Part print with two shaded views. Sizes in mm from the minimum x, y, z corner. A direction names the side the tool comes from. Give positions to 0.01 mm unless a question says otherwise; leave off trailing zeros. Order: outer loops, then holes, each group sorted by start corner. A loop starts at its lowest first (then second) coordinate and runs counter-clockwise, first axis right, second up. Notation, with made-up numbers: (48.25, -39.75) -> (107.25, -39.75) arc R24 ccw to (107.25, -1.75) -> close; hole circle Ø11 at (-26, 81). An arc over 180 degrees is marked (long way). Answer in a Markdown table with one row per item. Add a question column.
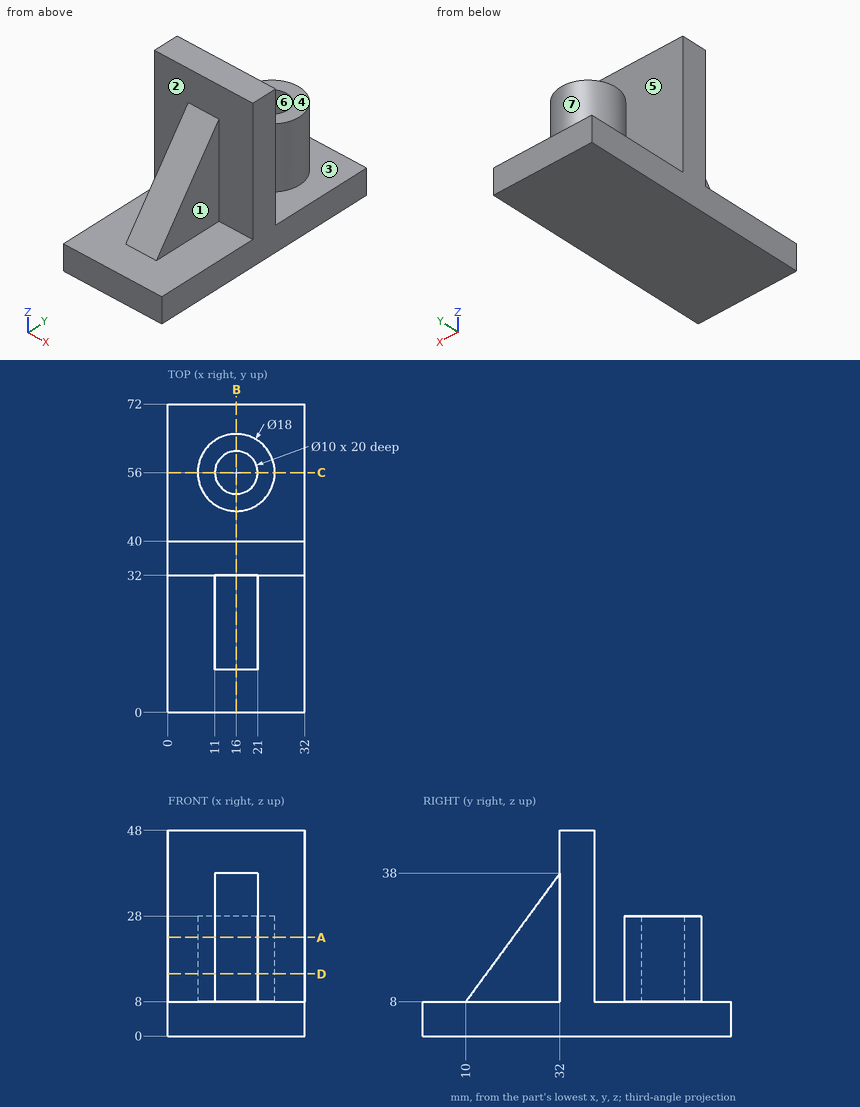
Item 1: Saw through at D-D on z = 14.5. List the corners of the cut face in (x, y), plus the area to 3 significant figures.
Item 2: Two-plate mould, pull along X, no slides. Class the marked faces 5, 6 and 7: pulls with the +X half, pulls with the -X half, needs draft (parallel to the pull), parting line crosses it, or undercut.
Item 3: Saw through at A-A on z = 23. List the corners of the cut face in (x, y).
Item 4: Saw through at B-B on x = 16. List the corners of the cut face in (y, z), plus the area to 3 significant figures.
Item 5: Pin check, flat tips, straight feed: pin 1 Ø2 at (x, z) = (28.5, 31) entering from -Y; pin 2 Ø4 at (x, z) = (17.5, 18) entering from +Y; pin 3 Ø8 at (x, z) = (20.5, 36) entering from +Y. Stop position of each tip, or through.
Item 6: Which spindle directions (+Z, -Z, +X, -X, +Y, -Y) get a long thin tool onto all of the face, cutting with end or side? Do the marked faces 1, 2, 3 and 4. Say none if no direction does.
Item 7: Saw through at C-C on y = 56. List the corners of the cut face in (x, z), plus the area to 3 significant figures.
Item 8: Wall check: line 1 (Y direction, x = 16, z = 22); line 2 (Z direction, x = 8, y = 61); line 3 (Y direction, x = 30.5, z = 25). Give the ranges that are in metal, low to high.
Evaluation:
| question | item | result |
|---|---|---|
| 1 | outline | (0, 32) -> (11, 32) -> (11, 14.77) -> (21, 14.77) -> (21, 32) -> (32, 32) -> (32, 40) -> (0, 40) -> close; circle Ø18 at (16, 56); hole circle Ø10 at (16, 56) |
| 1 | area | 604 mm2 |
| 2 | face 5 | needs draft |
| 2 | face 6 | undercut |
| 2 | face 7 | parting line crosses it |
| 3 | outline | (0, 32) -> (11, 32) -> (11, 21) -> (21, 21) -> (21, 32) -> (32, 32) -> (32, 40) -> (0, 40) -> close; circle Ø18 at (16, 56); hole circle Ø10 at (16, 56) |
| 4 | outline | (0, 0) -> (72, 0) -> (72, 8) -> (65, 8) -> (65, 28) -> (61, 28) -> (61, 8) -> (51, 8) -> (51, 28) -> (47, 28) -> (47, 8) -> (40, 8) -> (40, 48) -> (32, 48) -> (32, 38) -> (10, 8) -> (0, 8) -> close |
| 4 | area | 1,390 mm2 |
| 5 | pin 1 | stops at y = 32 |
| 5 | pin 2 | stops at y = 65 |
| 5 | pin 3 | stops at y = 40 |
| 6 | face 1 | +Z, +X, -Y |
| 6 | face 2 | +Z, -Y |
| 6 | face 3 | +Z |
| 6 | face 4 | +Z, +X, -X, +Y |
| 7 | outline | (0, 0) -> (32, 0) -> (32, 8) -> (25, 8) -> (25, 28) -> (21, 28) -> (21, 8) -> (11, 8) -> (11, 28) -> (7, 28) -> (7, 8) -> (0, 8) -> close |
| 7 | area | 416 mm2 |
| 8 | line 1 | y = 20.27 to 40, 47 to 51, 61 to 65 |
| 8 | line 2 | z = 0 to 8 |
| 8 | line 3 | y = 32 to 40 |
